from build123d import *

# Parameters (mm, degrees)
SKETCH1_W           = 118
SKETCH1_H           = 108
BOSS_EXTRUDE1_DEPTH = 4
SKETCH2_W           = 118
SKETCH2_H           = 108
SKETCH2_W_2         = 110
SKETCH2_H_2         = 100
BOSS_EXTRUDE2_DEPTH = 70
SKETCH3_W           = 80
SKETCH3_H           = 15
CUT_EXTRUDE1_DEPTH  = 4
SKETCH4_W           = 45
SKETCH4_H           = 15
CUT_EXTRUDE2_DEPTH  = 4
FILLET1_R           = 2


with BuildPart() as part:
    # Sketch1 → Boss-Extrude1 (new body)
    with BuildSketch(Plane(origin=(0, 0, 0), x_dir=(1, 0, 0), z_dir=(0, 1, 0))):
        with Locations((59, 54)):
            Rectangle(SKETCH1_W, SKETCH1_H)
    extrude(amount=BOSS_EXTRUDE1_DEPTH)

    # Sketch2 → Boss-Extrude2 (add)
    with BuildSketch(Plane(origin=(0, 4, 0), x_dir=(1, 0, 0), z_dir=(0, 1, 0))):
        with Locations((59, 54)):
            Rectangle(SKETCH2_W, SKETCH2_H)
        with Locations((59, 54)):
            Rectangle(SKETCH2_W_2, SKETCH2_H_2, mode=Mode.SUBTRACT)
    extrude(amount=BOSS_EXTRUDE2_DEPTH)

    # Sketch3 → Cut-Extrude1 (cut)
    with BuildSketch(Plane.ZY):
        with Locations((-54, 31.5)):
            Rectangle(SKETCH3_W, SKETCH3_H)
    extrude(amount=-CUT_EXTRUDE1_DEPTH, mode=Mode.SUBTRACT)

    # Sketch4 → Cut-Extrude2 (cut)
    with BuildSketch(Plane.XY):
        with Locations((91.5, 11.5)):
            Rectangle(SKETCH4_W, SKETCH4_H)
    extrude(amount=-CUT_EXTRUDE2_DEPTH, mode=Mode.SUBTRACT)

    # Fillet1
    fillet1_edges = [part.edges().sort_by_distance(p)[0] for p in [
        (0, 37, -108),
        (118, 37, -108),
        (118, 37, 0),
        (0, 37, 0),
    ]]
    fillet(fillet1_edges, radius=FILLET1_R)


solid = part.part
Work out the finished part from the listing and answer in its coordinate system (mm). A direction names the side the tool comes from. Coordinates: 2 decimals unless noted, no trailing zeros. Loops run counter-clockwise (first coordinate to the right, second up) from the corner with the lowest first, then second, coordinate; pieces in that order, holes last. Notation, with made-up numbers: M -15,-32 L 21,-32 A10 cw 21,-18 Z; hole C 69,38 d2. An arc over 180 degrees is marked long. Answer in a Markdown table with one row per item. Add a question column.
1. Find section C-C, the plane z = -55.5. Write down the section's boundary in (x, y).
2. A flat-ended cylindrical pin translates along its axis: P1, Ø5, axis at x = 66, z = -21.5, coming from the +Y side. Find the tip coordinate at first contact, or state that the pin passes through.
3. Consider L1, parallel to X at y = 19, z = -29; L2, parallel to Z at x = 100, y = 52; L3, parallel to Y at x = 31, z = -27. Determine where each line is inside the solid, lowest interval first.
4. Find section D-D, the plane y = 5.5. Write down the section's boundary in (x, z), then the cut area to 3 significant figures.
5. Find section B-B, the plane y = 67.5. Write down the section's boundary in (x, z).
6. A tool of negligible diameter and unlimited length cuts with its end or side. For faces 1 (the flat face through (2, 31, -94)), 2 (the flat face through (91, 19, -2)), 3 (the flat face through (58, 39, -4)), from which of +Z, -Z, +X, -X, +Y, -Y can it reach the whole face along a straight path? Write none if from no direction.
7. The mould has two halves that part along Y. Classify faces 4 (the flat face through (58, 39, -104)), 5 (the flat face through (2, 39, -55)), 6 (the flat face through (54, 74, -2)): pulls with the +Y half, pulls with the -Y half, needs draft (parallel to the pull), parting line crosses it, or undercut.
8. Find section A-A, the plane x = 101.5. Write down the section's boundary in (y, z).
Reported:
| question | item | result |
|---|---|---|
| 1 | outline | M 0,0 L 118,0 L 118,74 L 114,74 L 114,4 L 4,4 L 4,24 L 0,24 Z; M 0,39 L 4,39 L 4,74 L 0,74 Z |
| 2 | P1 | stops at y = 4 |
| 3 | L1 | x = 0 to 4, 114 to 118 |
| 3 | L2 | z = -108 to -104, -4 to 0 |
| 3 | L3 | y = 0 to 4 |
| 4 | outline | M 0,-106 A2 ccw 2,-108 L 116,-108 A2 ccw 118,-106 L 118,-2 A2 ccw 116,0 L 114,0 L 114,-104 L 4,-104 L 4,-4 L 69,-4 L 69,0 L 2,0 A2 ccw 0,-2 Z |
| 4 | area | 1,560 mm^2 |
| 5 | outline | M 0,-106 A2 ccw 2,-108 L 116,-108 A2 ccw 118,-106 L 118,-2 A2 ccw 116,0 L 2,0 A2 ccw 0,-2 Z; hole M 4,-104 L 114,-104 L 114,-4 L 4,-4 Z |
| 6 | face 1 | -X |
| 6 | face 2 | +Z |
| 6 | face 3 | +Y |
| 7 | face 4 | needs draft |
| 7 | face 5 | undercut |
| 7 | face 6 | pulls with the +Y half |
| 8 | outline | M 0,-108 L 74,-108 L 74,-104 L 4,-104 L 4,0 L 0,0 Z; M 19,-4 L 74,-4 L 74,0 L 19,0 Z |
